```python
from build123d import *

# Parameters (mm, degrees)
F0_W      = 121.92
F0_H      = 107.95
F1_DEPTH  = 38.1
F2_W      = 101.854
F2_H      = 101.854
F3_DEPTH  = 30.48
F5_DEPTH  = 25.4
F7_DEPTH  = 106.68
F8_W      = 121.92
F8_H      = 16.3267194241
F9_DEPTH  = 25.4
F10_DEPTH = 25.4


with BuildPart() as f1:
    # F0 (on Top) → F1 (new body)
    with BuildSketch(Plane.XY):
        Rectangle(F0_W, F0_H)
    extrude(amount=F1_DEPTH)

    # F2 (on face) → F3 (cut)
    with BuildSketch(Plane.XY.offset(38.1)):
        Rectangle(F2_W, F2_H)
    extrude(amount=-F3_DEPTH, mode=Mode.SUBTRACT)

    # F4 (on face) → F5 (cut)
    with BuildSketch(Plane(origin=(0, 0, 0), x_dir=(1, 0, 0), z_dir=(0, 0, -1))):
        with BuildLine():
            Line((-6.35, 26.193887236), (-6.35, 38.8158181091))
            ThreePointArc((-6.35, 38.8158181091), (-27.8117801972, 27.8117801972), (-38.8158181091, 6.35))
            Line((-38.8158181091, 6.35), (-26.193887236, 6.35))
            ThreePointArc((-26.193887236, 6.35), (-19.0583607445, 19.0583607445), (-6.35, 26.193887236))
        make_face()
        with BuildLine():
            Line((-26.193887236, -6.35), (-38.8158181091, -6.35))
            ThreePointArc((-38.8158181091, -6.35), (-27.8117801972, -27.8117801972), (-6.35, -38.8158181091))
            Line((-6.35, -38.8158181091), (-6.35, -26.193887236))
            ThreePointArc((-6.35, -26.193887236), (-19.0583607445, -19.0583607445), (-26.193887236, -6.35))
        make_face()
        with BuildLine():
            ThreePointArc((38.8158181091, 6.35), (27.8117801972, 27.8117801972), (6.35, 38.8158181091))
            Line((6.35, 38.8158181091), (6.35, 26.193887236))
            ThreePointArc((6.35, 26.193887236), (19.0583607445, 19.0583607445), (26.193887236, 6.35))
            Line((26.193887236, 6.35), (38.8158181091, 6.35))
        make_face()
        with BuildLine():
            ThreePointArc((26.193887236, -6.35), (19.0583607445, -19.0583607445), (6.35, -26.193887236))
            Line((6.35, -26.193887236), (6.35, -38.8158181091))
            ThreePointArc((6.35, -38.8158181091), (27.8117801972, -27.8117801972), (38.8158181091, -6.35))
            Line((38.8158181091, -6.35), (26.193887236, -6.35))
        make_face()
    extrude(amount=-F5_DEPTH, mode=Mode.SUBTRACT)

    # F6 (on face) → F7 (cut)
    with BuildSketch(Plane(origin=(0, 53.975, 0), x_dir=(-1, 0, 0), z_dir=(0, 1, 0))):
        Polygon((60.96, 15.748), (60.96, 38.1), (-60.96, 38.1), (-60.96, 15.748), (-51.308, 15.748), (-51.308, 10.668), (-53.848, 10.668), (-53.848, 5.08), (53.848, 5.08), (53.848, 10.668), (51.054, 10.668), (51.054, 15.748), align=None)
    extrude(amount=-F7_DEPTH, mode=Mode.SUBTRACT)

    # F8 (on face) → F9 (cut)
    with BuildSketch(Plane(origin=(0, -52.705, 0), x_dir=(-1, 0, 0), z_dir=(0, 1, 0))):
        with Locations((0, 29.9366402879)):
            Rectangle(F8_W, F8_H)
    extrude(amount=-F9_DEPTH, mode=Mode.SUBTRACT)

    # F4 (on face) → F10 (cut)
    with BuildSketch(Plane(origin=(0, 0, 0), x_dir=(1, 0, 0), z_dir=(0, 0, -1))):
        with BuildLine():
            Line((-6.35, 26.193887236), (-6.35, 38.8158181091))
            ThreePointArc((-6.35, 38.8158181091), (-27.8117801972, 27.8117801972), (-38.8158181091, 6.35))
            Line((-38.8158181091, 6.35), (-26.193887236, 6.35))
            ThreePointArc((-26.193887236, 6.35), (-19.0583607445, 19.0583607445), (-6.35, 26.193887236))
        make_face()
        with BuildLine():
            Line((-26.193887236, -6.35), (-38.8158181091, -6.35))
            ThreePointArc((-38.8158181091, -6.35), (-27.8117801972, -27.8117801972), (-6.35, -38.8158181091))
            Line((-6.35, -38.8158181091), (-6.35, -26.193887236))
            ThreePointArc((-6.35, -26.193887236), (-19.0583607445, -19.0583607445), (-26.193887236, -6.35))
        make_face()
        with BuildLine():
            ThreePointArc((38.8158181091, 6.35), (27.8117801972, 27.8117801972), (6.35, 38.8158181091))
            Line((6.35, 38.8158181091), (6.35, 26.193887236))
            ThreePointArc((6.35, 26.193887236), (19.0583607445, 19.0583607445), (26.193887236, 6.35))
            Line((26.193887236, 6.35), (38.8158181091, 6.35))
        make_face()
        with BuildLine():
            ThreePointArc((26.193887236, -6.35), (19.0583607445, -19.0583607445), (6.35, -26.193887236))
            Line((6.35, -26.193887236), (6.35, -38.8158181091))
            ThreePointArc((6.35, -38.8158181091), (27.8117801972, -27.8117801972), (38.8158181091, -6.35))
            Line((38.8158181091, -6.35), (26.193887236, -6.35))
        make_face()
    extrude(amount=-F10_DEPTH, mode=Mode.SUBTRACT)


solid = f1.part
```
Geometry check sheet. Reference: the model listing, model coordinates, mm. A direction names the side the tool comes from. Coordinates: 2 decimals unless noted, no trailing zeros. Loops run counter-clockwise (first coordinate to the right, second up) from the corner with the lowest first, then second, coordinate; pieces in that order, holes last.
Item 1: Sectioned sample at B-B, the plane x = -28. Record the boundary of the cut face in (y, z) (3 decimals), then the cut area to 3 significant figures.
Item 2: Go/stop test with flat-tipped pins: pin 1 Ø1.5 at (x, y) = (-13.5, 10) entering from +Z; pin 2 Ø2 at (x, y) = (36, -8) entering from +Z (1 decimal); pin 3 Ø8 at (x, y) = (-54, -17) entering from +Z; pin 4 Ø2 at (x, z) = (23, 13.5) entering from +Y (3 decimals). Record where each tip stops, or that it passes through.
Item 3: Access from +Z, -Z, +X, -X, +Y, -Y to the whole of each face (thin tool, end or side, straight path). Record for faces 1 (the face through (-53.848, 1, 8)), 2 (the face through (-56, 1, 15.748)), 3 (the face through (-32, 6.35, 3)), 4 (the face through (-51.054, 1, 13)).
Item 4: Sectioned sample at D-D, the plane z = 9. Record the boundary of the cut face in (x, y) (3 decimals), then the cut area to 3 significant figures.
Item 5: Thickness scan on line 1 (X direction, y = 49.5, z = 9.5); line 2 (X direction, y = 22, z = 1); line 3 (Z direction, x = -51.5, y = -8). Record the ranges inside material, lowest first.
Item 6: Release check for a two-part mould opening along X. For faces 5 (the face through (60.96, -1, 8)), 6 (the face through (51.308, 1, 13)), 7 (the face through (-1, -53.975, 11)) record: released by +X, released by -X, zero draft, split by the parting line, or undercut.
Item 7: Sectioned sample at C-C, the plane y = 35. Record the boundary of the cut face in (x, z).
Item 8: Sectioned sample at A-A, the plane z = 2.25. Record the boundary of the cut face in (x, y) (3 decimals), then the cut area to 3 significant figures.
Check result:
1. outline: (-53.975, 0) - (-27.622, 0) - (-27.622, 5.08) - (-52.705, 5.08) - (-52.705, 21.773) - (-53.975, 21.773) - close; (-6.35, 0) - (6.35, 0) - (6.35, 5.08) - (-6.35, 5.08) - close; (27.622, 0) - (53.975, 0) - (53.975, 5.08) - (27.622, 5.08) - close
1. area: 353 mm2
2. pin 1: stops at z = 5.08
2. pin 2: passes through
2. pin 3: stops at z = 15.75
2. pin 4: stops at y = -52.705
3. face 1: +Y
3. face 2: +Z, +X, -X, +Y
3. face 3: +Z, -Z
3. face 4: +Z, +Y
4. outline: (-60.96, -53.975) - (60.96, -53.975) - (60.96, 53.975) - (53.848, 53.975) - (53.848, -52.705) - (-53.848, -52.705) - (-53.848, 53.975) - (-60.96, 53.975) - close
4. area: 1,670 mm2
5. line 1: x = -60.96 to -53.85, 53.85 to 60.96
5. line 2: x = -60.96 to -32.6, -15.57 to 15.57, 32.6 to 60.96
5. line 3: z = 0 to 5.08, 10.67 to 15.75
6. face 5: released by +X
6. face 6: undercut
6. face 7: zero draft
7. outline: (-60.96, 0) - (-17.94, 0) - (-17.94, 5.08) - (-53.85, 5.08) - (-53.85, 10.67) - (-51.05, 10.67) - (-51.05, 15.75) - (-60.96, 15.75) - close; (-6.35, 0) - (6.35, 0) - (6.35, 5.08) - (-6.35, 5.08) - close; (17.94, 0) - (60.96, 0) - (60.96, 15.75) - (51.31, 15.75) - (51.31, 10.67) - (53.85, 10.67) - (53.85, 5.08) - (17.94, 5.08) - close
8. outline: (-60.96, -53.975) - (60.96, -53.975) - (60.96, 53.975) - (-60.96, 53.975) - close; hole (-38.816, -6.35) arc R39.332 ccw to (-6.35, -38.816) - (-6.35, -26.194) arc R26.953 cw to (-26.194, -6.35) - close; hole (-38.816, 6.35) - (-26.194, 6.35) arc R26.953 cw to (-6.35, 26.194) - (-6.35, 38.816) arc R39.332 ccw to start; hole (6.35, -38.816) arc R39.332 ccw to (38.816, -6.35) - (26.194, -6.35) arc R26.953 cw to (6.35, -26.194) - close; hole (6.35, 26.194) arc R26.953 cw to (26.194, 6.35) - (38.816, 6.35) arc R39.332 ccw to (6.35, 38.816) - close
8. area: 11,200 mm2
